For this review, take the finished solid that the model builds, in its own axes (mm). A direction names the side the tool comes from. Give positions to 0.01 mm unless a question says otherwise; leave off trailing zeros. Write each loop counter-clockwise with the first axis right and the second up, starting at its lowest first coordinate (ties: lowest second). Pieces come first, ordered by that corner, then holes.
from build123d import *

# Parameters (mm, degrees)
F0_W     = 127
F0_H     = 228.6
F1_DEPTH = 17.4625
F3_D     = 11.50874
F4_W     = 400.05
F4_H     = 12.7
F5_DEPTH = 152.4
F7_DEPTH = 190.501
F8_SIZE  = 12.7


with BuildPart() as f1:
    # F0 (on Top) → F1 (new body)
    with BuildSketch(Plane.XY):
        Rectangle(F0_W, F0_H)
    extrude(amount=F1_DEPTH)

    # F3 (through all)
    with Locations(Plane.XY.offset(17.4625)):
        with Locations((-44.45, 95.25), (44.45, 95.25), (44.45, -95.25), (-44.45, -95.25)):
            Hole(F3_D / 2)

    # F4 (on face) → F5 (join)
    with BuildSketch(Plane(origin=(0, 0, 0), x_dir=(1, 0, 0), z_dir=(0, 0, -1))):
        with Locations((-149.225, -69.85)):
            Rectangle(F4_W, F4_H)
    extrude(amount=F5_DEPTH)

    # F6 (on face) → F7 (cut, through all)
    with BuildSketch(Plane(origin=(0, 76.2, 0), x_dir=(-1, 0, 0), z_dir=(0, 1, 0))):
        Polygon((-50.8, -12.7), (-50.8, -152.4), (298.45, -152.4), align=None)
    extrude(amount=-F7_DEPTH, mode=Mode.SUBTRACT)

    # F8
    f8_edges = [f1.edges().sort_by_distance(p)[0] for p in [
        (-349.25, 69.85, 0),
    ]]
    chamfer(f8_edges, length=F8_SIZE)

    # F9: F1 across plane


with BuildPart() as f1_1:
    add(f1.part)
    add(f1.part.mirror(Plane.XZ))


solid = f1_1.part
(1) We need section C-C (x = -110.5). Write out the cut boundary in (y, z), and give its area (3 significant figures).
(2) Clearance check with flat-ended pins moving along their axes: pin 1 Ø5 at (x, z) = (-277.5, -120.5) entering from +Y; pin 2 Ø10 at (x, z) = (-84, -68) entering from -Y; pin 3 Ø8.5 at (y, z) = (-42.5, 12) entering from -X. State where each tip first meets the part, or that it passes through.
(3) We need section A-A (z = -104). Write out the cut boundary in (x, y).
(4) We need section B-B (x = -44.45). Write out the cut boundary in (y, z), and give its area (3 significant figures).
(5) The part is to be moulded in two halves that separate along X. For faces 5 (the flat face through (-324, 70, -152.4)), 6 (the flat face through (50.8, -70, -6)), 7 (the cylindrical face through (41.795, -100.355, 8.609)), 8 (the cylindrical face through (38.96, 96.98, 8.61)), say which applies: +X half, -X half, draft (parallel to the pull), parting line (faces both ways), or undercut.
(6) For L1, parallel to Y at x = 44.45, z = 11; L2, parallel to Y at x = -77, z = -47; L3, parallel to Z at x = -59.5, y = -80, list the stretches that pass through material, from the lowest coordinate up.
(7) We need section D-D (y = 95.25). Write out the cut boundary in (x, z).
(8) Tool access review of faces 1 (the flat face through (50.8, 70, -6)), 2 (the flat face through (-196, -76.2, -58)), 3 (the flat face through (-196, 76.2, -58)), 4 (the flat face through (-196, -63.5, -58)): name each direction out of +Z, -Z, +X, -X, +Y, -Y from which nothing blocks a thin tool from reaching the whole face with its end or side.
The answers:
1. outline: (-76.2, -77.22) - (-63.5, -77.22) - (-63.5, 0) - (-76.2, 0) - close; (63.5, -77.22) - (76.2, -77.22) - (76.2, 0) - (63.5, 0) - close
1. area: 1,960 mm2
2. pin 1: stops at y = 76.2
2. pin 2: stops at y = -76.2
2. pin 3: stops at x = -63.5
3. outline: (-349.25, -76.2) - (-177.45, -76.2) - (-177.45, -63.5) - (-349.25, -63.5) - close; (-349.25, 63.5) - (-177.45, 63.5) - (-177.45, 76.2) - (-349.25, 76.2) - close
4. outline: (-114.3, 0) - (-101, 0) - (-101, 17.46) - (-114.3, 17.46) - close; (-89.5, 0) - (-76.2, 0) - (-76.2, -50.8) - (-63.5, -50.8) - (-63.5, 0) - (63.5, 0) - (63.5, -50.8) - (76.2, -50.8) - (76.2, 0) - (89.5, 0) - (89.5, 17.46) - (-89.5, 17.46) - close; (101, 0) - (114.3, 0) - (114.3, 17.46) - (101, 17.46) - close
4. area: 4,880 mm2
5. face 5: draft
5. face 6: +X half
5. face 7: undercut
5. face 8: undercut
6. L1: y = -114.3 to -101, -89.5 to 89.5, 101 to 114.3
6. L2: y = -76.2 to -63.5, 63.5 to 76.2
6. L3: z = 0 to 17.46
7. outline: (-63.5, 0) - (-50.2, 0) - (-50.2, 17.46) - (-63.5, 17.46) - close; (-38.7, 0) - (38.7, 0) - (38.7, 17.46) - (-38.7, 17.46) - close; (50.2, 0) - (63.5, 0) - (63.5, 17.46) - (50.2, 17.46) - close
8. face 1: -Z, +X, +Y, -Y
8. face 2: -Z, +X, -X, -Y
8. face 3: -Z, +X, -X, +Y
8. face 4: -Z, +X, -X
